from build123d import *

# Parameters (mm, degrees)
SKETCH_1_W               = 240
SKETCH_1_H               = 180
EXTRUDE_1_DEPTH          = 2
SKETCH_3_R               = 2.1
CUT_EXTRUDE_2_DEPTH      = 10
CUT_EXTRUDE_3_DEPTH      = 151.013332741
CUT_EXTRUDE_3_DEPTH_BACK = 10
SKETCH_4_R               = 1.6
SKETCH_4_R_2             = 1.25
SKETCH_4_R_3             = 1.75
SKETCH_5_R               = 1.6
CUT_EXTRUDE_4_DEPTH      = 10
SKETCH_6_W               = 110
SKETCH_6_H               = 60
SKETCH_6_W_2             = 35
SKETCH_6_H_2             = 50
SKETCH_6_W_3             = 20
SKETCH_6_H_3             = 20
SKETCH_6_W_4             = 45
SKETCH_6_H_4             = 31
SKETCH_6_W_5             = 95
SKETCH_6_H_5             = 10
CUT_EXTRUDE_5_DEPTH      = 10
SKETCH_7_W               = 52
SKETCH_7_H               = 29
CUT_EXTRUDE_6_DEPTH      = 10
FILLET_1_R               = 3
CHAMFER_1_SIZE           = 3


with BuildPart() as part:
    # Sketch 1 → Extrude 1 (new body)
    with BuildSketch(Plane(origin=(0, 0, 0), x_dir=(1, 0, 0), z_dir=(0, 1, 0))):
        Rectangle(SKETCH_1_W, SKETCH_1_H)
    extrude(amount=EXTRUDE_1_DEPTH)

    # Sketch 3 → Cut-Extrude 2 (cut)
    with BuildSketch(Plane(origin=(0, 2, 0), x_dir=(1, 0, 0), z_dir=(0, 1, 0))):
        with Locations(Location((-110, 80, 0), (0, 0, 270))):
            Circle(SKETCH_3_R)
        with Locations(Location((-110, 0, 0), (0, 0, 270))):
            Circle(SKETCH_3_R)
        with Locations(Location((-110, -80, 0), (0, 0, 270))):
            Circle(SKETCH_3_R)
        with Locations(Location((110, -80, 0), (0, 0, 270))):
            Circle(SKETCH_3_R)
        with Locations(Location((110, 0, 0), (0, 0, 270))):
            Circle(SKETCH_3_R)
        with Locations(Location((110, 80, 0), (0, 0, 270))):
            Circle(SKETCH_3_R)
    extrude(amount=-CUT_EXTRUDE_2_DEPTH, mode=Mode.SUBTRACT)

    # Sketch 4 → Cut-Extrude 3 (cut, two sides: drawn at the far end of the back side and taken through both)
    with BuildSketch(Plane(origin=(0, 2, 0), x_dir=(1, 0, 0), z_dir=(0, 1, 0)).offset(-CUT_EXTRUDE_3_DEPTH_BACK)):
        with Locations(Location((40, 80, 0), (0, 0, 90))):
            Circle(SKETCH_4_R)
        with Locations(Location((95, 80, 0), (0, 0, 90))):
            Circle(SKETCH_4_R)
        with Locations(Location((40, 39, 0), (0, 0, 90))):
            Circle(SKETCH_4_R)
        with Locations(Location((95, 39, 0), (0, 0, 90))):
            Circle(SKETCH_4_R)
        with Locations(Location((65, 14, 0), (0, 0, 90))):
            Circle(SKETCH_4_R_2)
        with Locations(Location((95, 14, 0), (0, 0, 90))):
            Circle(SKETCH_4_R_2)
        with Locations(Location((95, -16, 0), (0, 0, 90))):
            Circle(SKETCH_4_R_2)
        with Locations(Location((65, -16, 0), (0, 0, 90))):
            Circle(SKETCH_4_R_2)
        with Locations(Location((95, -31, 0), (0, 0, 90))):
            Circle(SKETCH_4_R_2)
        with Locations(Location((65, -31, 0), (0, 0, 90))):
            Circle(SKETCH_4_R_2)
        with Locations(Location((65, -61, 0), (0, 0, 90))):
            Circle(SKETCH_4_R_2)
        with Locations(Location((95, -61, 0), (0, 0, 90))):
            Circle(SKETCH_4_R_2)
        with Locations(Location((50, -31, 0), (0, 0, 90))):
            Circle(SKETCH_4_R_2)
        with Locations(Location((20, -31, 0), (0, 0, 90))):
            Circle(SKETCH_4_R_2)
        with Locations(Location((20, -61, 0), (0, 0, 90))):
            Circle(SKETCH_4_R_2)
        with Locations(Location((50, -61, 0), (0, 0, 90))):
            Circle(SKETCH_4_R_2)
        with Locations(Location((-95, 50, 0), (0, 0, 90))):
            Circle(SKETCH_4_R_3)
        with Locations(Location((-95, 70, 0), (0, 0, 90))):
            Circle(SKETCH_4_R_3)
        with Locations(Location((10, 70, 0), (0, 0, 90))):
            Circle(SKETCH_4_R_3)
        with Locations(Location((10, 50, 0), (0, 0, 90))):
            Circle(SKETCH_4_R_3)
    extrude(amount=CUT_EXTRUDE_3_DEPTH + CUT_EXTRUDE_3_DEPTH_BACK, mode=Mode.SUBTRACT)

    # Sketch 5 → Cut-Extrude 4 (cut)
    with BuildSketch(Plane(origin=(0, 2, 0), x_dir=(1, 0, 0), z_dir=(0, 1, 0))):
        with Locations(Location((-62.5, -65, 0), (0, 0, 270))):
            Circle(SKETCH_5_R)
        with Locations(Location((-77.5, -65, 0), (0, 0, 270))):
            Circle(SKETCH_5_R)
        with Locations(Location((-50, -75, 0), (0, 0, 270))):
            Circle(SKETCH_5_R)
        with Locations(Location((-90, -75, 0), (0, 0, 270))):
            Circle(SKETCH_5_R)
        with Locations(Location((-90, -55, 0), (0, 0, 270))):
            Circle(SKETCH_5_R)
        with Locations(Location((-50, -55, 0), (0, 0, 270))):
            Circle(SKETCH_5_R)
    extrude(amount=-CUT_EXTRUDE_4_DEPTH, mode=Mode.SUBTRACT)

    # Sketch 6 → Cut-Extrude 5 (cut)
    with BuildSketch(Plane(origin=(0, 2, 0), x_dir=(1, 0, 0), z_dir=(0, 1, 0))):
        with Locations((-45, -15)):
            Rectangle(SKETCH_6_W, SKETCH_6_H)
        with Locations((37.5, 4)):
            Rectangle(SKETCH_6_W_2, SKETCH_6_H_2)
        with Locations((80, -1)):
            Rectangle(SKETCH_6_W_3, SKETCH_6_H_3)
        with Locations((80, -46)):
            Rectangle(SKETCH_6_W_3, SKETCH_6_H_3)
        with Locations((35, -46)):
            Rectangle(SKETCH_6_W_3, SKETCH_6_H_3)
        with Locations((67.5, 59.5)):
            Rectangle(SKETCH_6_W_4, SKETCH_6_H_4)
        with Locations((-42.5, 60)):
            Rectangle(SKETCH_6_W_5, SKETCH_6_H_5)
    extrude(amount=-CUT_EXTRUDE_5_DEPTH, mode=Mode.SUBTRACT)

    # Sketch 7 → Cut-Extrude 6 (cut)
    with BuildSketch(Plane(origin=(0, 2, 0), x_dir=(1, 0, 0), z_dir=(0, 1, 0))):
        with Locations((-14, -67.5)):
            Rectangle(SKETCH_7_W, SKETCH_7_H)
    extrude(amount=-CUT_EXTRUDE_6_DEPTH, mode=Mode.SUBTRACT)

    # Fillet 1
    fillet_1_edges = [part.edges().sort_by_distance(p)[0] for p in [
        (-90, 1, -65),
        (5, 1, -65),
        (5, 1, -55),
        (-90, 1, -55),
        (45, 1, -75),
        (90, 1, -75),
        (90, 1, -44),
        (45, 1, -44),
        (25, 1, 36),
        (45, 1, 36),
        (45, 1, 56),
        (25, 1, 56),
        (70, 1, 36),
        (90, 1, 36),
        (90, 1, 56),
        (70, 1, 56),
        (70, 1, -9),
        (90, 1, -9),
        (90, 1, 11),
        (70, 1, 11),
        (55, 1, -29),
        (55, 1, 21),
        (20, 1, 21),
        (20, 1, -29),
        (10, 1, -15),
        (10, 1, 45),
        (-100, 1, 45),
        (-100, 1, -15),
        (-40, 1, 82),
        (-40, 1, 53),
        (12, 1, 53),
        (12, 1, 82),
    ]]
    fillet(fillet_1_edges, radius=FILLET_1_R)

    # Chamfer 1
    chamfer_1_edges = [part.edges().sort_by_distance(p)[0] for p in [
        (120, 1, 90),
        (-120, 1, 90),
        (-120, 1, -90),
        (120, 1, -90),
    ]]
    chamfer(chamfer_1_edges, length=CHAMFER_1_SIZE)


solid = part.part
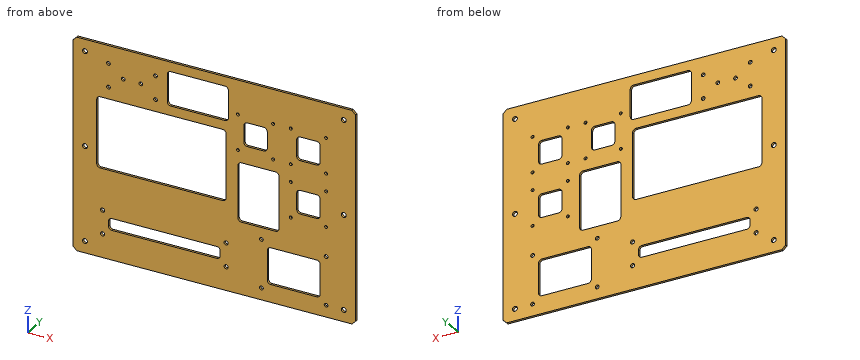
Verification items for the finished model (mm, model axes). Coordinates: 2 decimals unless noted, no trailing zeros. Write each loop counter-clockwise with the first axis right and the second up, starting at its lowest first coordinate (ties: lowest second). Pieces come first, ordered by that corner, then holes. Notation, with made-up numbers: M -10,18.5 L 20,18.5 A33 cw 20,57.5 Z; hole C 7,38 d3. An arc over 180 degrees is marked long. Use a Markdown table: item, result.
Q1. Sectioned sample at C-C, the plane y = 1.5. Count the separate pieces of the cut face and the enclosed holes in it, plus the area to 3 significant figures.
Reply:
| item | result |
|---|---|
| separate pieces | 1 |
| enclosed holes | 40 |
| area | 29,600 mm² |
Q2. Sectioned sample at A-A, the plane x = -6. Record the boundary of the cut face in (y, z).
Reply:
| item | result |
|---|---|
| outline | M 0,-90 L 2,-90 L 2,-65 L 0,-65 Z; M 0,-55 L 2,-55 L 2,-15 L 0,-15 Z; M 0,45 L 2,45 L 2,53 L 0,53 Z; M 0,82 L 2,82 L 2,90 L 0,90 Z |
Q3. Sectioned sample at B-B, the plane z = -22. Record the boundary of the cut face in (x, y), plus the area to 3 significant figures.
Reply:
| item | result |
|---|---|
| outline | M -120,0 L 20,0 L 20,2 L -120,2 Z; M 55,0 L 120,0 L 120,2 L 55,2 Z |
| area | 410 mm² |
Q4. Thickness scan on line 1 (Z direction, x = 65, y = 0.55); line 2 (Z direction, x = -27.5, y = 1.7); line 3 (X direction, y = 0.85, z = -50). Record the ranges inside material, lowest first.
Reply:
| item | result |
|---|---|
| line 1 | z = -90 to -75, -44 to -15.25, -12.75 to 14.75, 17.25 to 29.75, 32.25 to 59.75, 62.25 to 90 |
| line 2 | z = -90 to -65, -55 to -15, 45 to 53, 82 to 90 |
| line 3 | x = -120 to -96.75, -93.25 to 8.25, 11.75 to 45, 90 to 120 |
